Here's how the part is built. I have some questions about the finished solid (model axes, mm). Face numbers are marked on the shaded views. A direction names the side the tool comes from. Round coordinates to 2 decimals unless told otherwise and drop trailing zeros. Loops run counter-clockwise (first coordinate to the right, second up) from the corner with the lowest first, then second, coordinate; pieces in that order, holes last. Notation, with made-up numbers: (-38.5, 28.25) -> (8.5, 28.25) arc R5 ccw to (8.5, 32.25) -> close; hole circle Ø7 at (39, 11). An arc over 180 degrees is marked (long way). One line per item, written item: value. Start each with the question number.
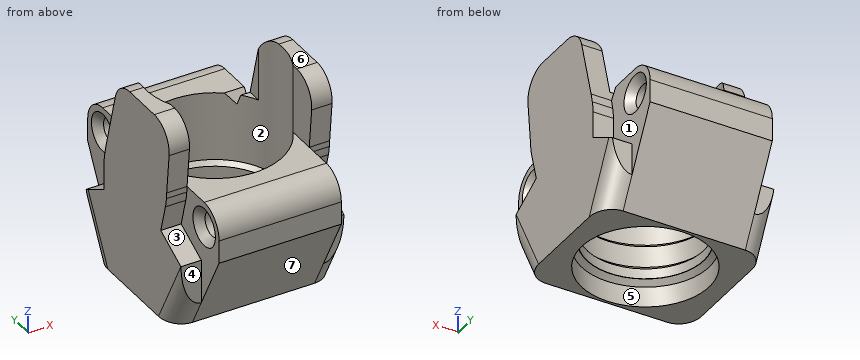
```python
from build123d import *

# Parameters (mm, degrees)
BOSS_EXTRUDE1_DEPTH           = 16
SKETCH2_W                     = 4
SKETCH2_H                     = 6.039060338
CUT_EXTRUDE1_DEPTH            = 49.391321349
FILLET1_R                     = 4
CUT_EXTRUDE2_DEPTH            = 4
SKETCH4_R                     = 12.5
CUT_EXTRUDE3_DEPTH            = 5
SKETCH5_R                     = 11.435
CUT_EXTRUDE4_DEPTH            = 45.34771704
CUT_EXTRUDE5_START            = -2
SKETCH7_R                     = 12.5
CUT_EXTRUDE5_DEPTH            = 43.347717155
CUT_EXTRUDE6_START            = 5
SKETCH8_R                     = 13.322
CUT_EXTRUDE6_DEPTH            = 38.786914196
CHAMFER5_SIZE                 = 1
SKETCH9_W                     = 24
SKETCH9_H                     = 20
CUT_EXTRUDE7_DEPTH            = 59.111966759
CSK_FOR_M4_SFHCS1_D           = 4.5
CSK_FOR_M4_SFHCS1_CSINK_D     = 7.5
CSK_FOR_M4_SFHCS1_CSINK_ANGLE = 90


with BuildPart() as part:
    # Sketch1 → Boss-Extrude1 (new, symmetric)
    with BuildSketch(Plane(origin=(0, 0, 0), x_dir=(0, 0, -1), z_dir=(1, 0, 0))):
        with BuildLine():
            Line((0, 13), (0, -13))
            Line((0, -13), (-17, -21.960950792))
            Line((-17, -21.960950792), (-21.5, -21.960950792))
            ThreePointArc((-21.5, -21.960950792), (-25.035533906, -20.496484698), (-26.5, -16.960950792))
            Line((-26.5, -16.960950792), (-26.5, -11.227190102))
            Line((-26.5, -11.227190102), (-34.5, -12.031216319))
            ThreePointArc((-34.5, -12.031216319), (-38.354100408, -10.76437729), (-39.999997516, -7.056278884))
            Line((-39.999997516, -7.056278884), (-39.999997516, 1.132402994))
            ThreePointArc((-39.999997516, 1.132402994), (-38.966764217, 4.176210139), (-36.294092741, 5.962032125))
            Line((-36.294092741, 5.962032125), (-24.512466398, 9.118909389))
            Line((-24.512466398, 9.118909389), (-26.5, 10.584515032))
            Line((-26.5, 10.584515032), (-26.5, 17.039060338))
            ThreePointArc((-26.5, 17.039060338), (-25.035533906, 20.574594244), (-21.5, 22.039060338))
            Line((-21.5, 22.039060338), (-17, 22.039060338))
            Line((-17, 22.039060338), (0, 13))
        make_face()
    extrude(amount=BOSS_EXTRUDE1_DEPTH, both=True)

    # Sketch2 → Cut-Extrude1 (cut, through all)
    with BuildSketch(Plane(origin=(0, 0, 0), x_dir=(-1, 0, 0), z_dir=(0, 0, -1))):
        with Locations((-14, 19.019530169)):
            Rectangle(SKETCH2_W, SKETCH2_H)
        with Locations((14, 19.019530169)):
            Rectangle(SKETCH2_W, SKETCH2_H)
        with Locations((14, -19.019530169)):
            Rectangle(SKETCH2_W, SKETCH2_H)
        with Locations((-14, -19.019530169)):
            Rectangle(SKETCH2_W, SKETCH2_H)
    extrude(amount=-CUT_EXTRUDE1_DEPTH, mode=Mode.SUBTRACT)

    # Fillet1
    fillet1_edges = [part.edges().sort_by_distance(p)[0] for p in [
        (16, -14.5, 2.845680173),
        (-16, -14.5, 2.845680173),
        (16, 14.5, 2.821089698),
        (-16, 14.5, 2.821089698),
    ]]
    fillet(fillet1_edges, radius=FILLET1_R)

    # Sketch3 → Cut-Extrude2 (cut)
    with BuildSketch(Plane.ZY.offset(16)):
        with BuildLine():
            Line((14.269532395, -16), (17.810147733, -9.256580566))
            Line((17.810147733, -9.256580566), (23.455857772, -10.805790893))
            ThreePointArc((23.455857772, -10.805790893), (24.367969512, -11.010765142), (25.295236814, -11.12966687))
            Line((25.295236814, -11.12966687), (26.5, -11.227190102))
            Line((26.5, -11.227190102), (26.5, -16))
            Line((26.5, -16), (14.269532395, -16))
        make_face()
        with BuildLine():
            Line((11.870259532, 16), (15.370259532, 9.753066737))
            Line((15.370259532, 9.753066737), (20.553734624, 9.753066737))
            ThreePointArc((20.553734624, 9.753066737), (21.64061559, 9.693825703), (22.714618956, 9.516804502))
            Line((22.714618956, 9.516804502), (24.512466398, 9.118909389))
            Line((24.512466398, 9.118909389), (26.5, 10.584515032))
            Line((26.5, 10.584515032), (26.5, 16))
            Line((26.5, 16), (11.870259532, 16))
        make_face()
    cut_extrude2 = extrude(amount=-CUT_EXTRUDE2_DEPTH, mode=Mode.SUBTRACT)

    # Mirror1: Cut-Extrude2 across plane
    add(cut_extrude2.mirror(Plane(origin=(0, 0, 0), x_dir=(0, 0, 1), z_dir=(1, 0, 0))), mode=Mode.SUBTRACT)

    # Sketch4 → Cut-Extrude3 (cut)
    with BuildSketch(Plane(origin=(0, 0, 0), x_dir=(-1, 0, 0), z_dir=(0, 0, -1))):
        with Locations(Location((0, 0, 0), (0, 0, 90))):
            Circle(SKETCH4_R)
    extrude(amount=-CUT_EXTRUDE3_DEPTH, mode=Mode.SUBTRACT)

    # Sketch5 → Cut-Extrude4 (cut, through all)
    with BuildSketch(Plane(origin=(0, 0, 5), x_dir=(-1, 0, 0), z_dir=(0, 0, -1))):
        with Locations(Location((0, 0, 0), (0, 0, 90))):
            Circle(SKETCH5_R)
    extrude(amount=-CUT_EXTRUDE4_DEPTH, mode=Mode.SUBTRACT)

    # Sketch7 → Cut-Extrude5 (cut, through all)
    with BuildSketch(Plane(origin=(0, 0, 5), x_dir=(-1, 0, 0), z_dir=(0, 0, -1)).offset(CUT_EXTRUDE5_START)):
        with Locations(Location((0, 0, 0), (0, 0, 90))):
            Circle(SKETCH7_R)
    extrude(amount=-CUT_EXTRUDE5_DEPTH, mode=Mode.SUBTRACT)

    # Sketch8 → Cut-Extrude6 (cut, through all)
    with BuildSketch(Plane.XY.offset(7).offset(CUT_EXTRUDE6_START)):
        with Locations(Location((0, 0, 0), (0, 0, 175.123832714))):
            Circle(SKETCH8_R)
    extrude(amount=CUT_EXTRUDE6_DEPTH, mode=Mode.SUBTRACT)

    # Chamfer5
    # the kernel refuses this chamfer: 1 mm, written as the material it adds along each edge
    with BuildSketch(Plane(origin=(0, 0, 7), x_dir=(0, 1, 0), z_dir=(-1, 0, 0))) as chamfer5_piece_1:
        Polygon((12.5 - CHAMFER5_SIZE, 0), (12.5, -CHAMFER5_SIZE), (12.5, 0), align=None)
    revolve(axis=Axis((0, 0, 7), (0, 0, -1)))
    with BuildSketch(Plane(origin=(0, 0, 5), x_dir=(0, 1, 0), z_dir=(-1, 0, 0))) as chamfer5_piece_2:
        Polygon((12.5, CHAMFER5_SIZE), (12.5 - CHAMFER5_SIZE, 0), (12.5, 0), align=None)
    revolve(axis=Axis((0, 0, 5), (0, 0, -1)))
    with BuildSketch(Plane(origin=(0, 0, 12), x_dir=(-0.9963807399610061, 0.08500247663896625, 0), z_dir=(0.08500247663896625, 0.9963807399610061, 0))) as chamfer5_piece_3_section:
        Polygon((13.322, CHAMFER5_SIZE), (13.322 - CHAMFER5_SIZE, 0), (13.322, 0), align=None)
    chamfer5_piece_3 = revolve(axis=Axis((0, 0, 12), (0, 0, 1)), mode=Mode.PRIVATE)
    chamfer5_piece_3 = chamfer5_piece_3 - Plane(origin=(0, 0, 12.578358266), x_dir=(0, 1, 0), z_dir=(0, 0, -1)) * Cylinder(12.5, 54, mode=Mode.PRIVATE)
    add(chamfer5_piece_3)

    # Sketch9 → Cut-Extrude7 (cut, through all)
    with BuildSketch(Plane(origin=(0, 17.039060338, 0), x_dir=(-1, 0, 0), z_dir=(0, 1, 0))):
        with Locations((0, 36.5)):
            Rectangle(SKETCH9_W, SKETCH9_H)
    extrude(amount=-CUT_EXTRUDE7_DEPTH, mode=Mode.SUBTRACT)

    # CSK for M4 SFHCS1 (through all)
    with Locations(Plane(origin=(12, 0, 0), x_dir=(0, 0, -1), z_dir=(1, 0, 0))):
        with Locations((-21.5, 17.039060338), (-21.5, -16.960950792)):
            csk_for_m4_sfhcs1 = CounterSinkHole(CSK_FOR_M4_SFHCS1_D / 2, CSK_FOR_M4_SFHCS1_CSINK_D / 2, counter_sink_angle=CSK_FOR_M4_SFHCS1_CSINK_ANGLE)

    # Mirror2: CSK for M4 SFHCS1 across plane
    add(csk_for_m4_sfhcs1.mirror(Plane(origin=(0, 0, 0), x_dir=(0, 0, 1), z_dir=(1, 0, 0))), mode=Mode.SUBTRACT)


solid = part.part
```
Q1. I want a section at A-A on x = 0. State how many separate pieces and enclosed holes the cut face has, plus the area to 3 significant figures.
Q2. I want a section at B-B on y = 0. Please give me the cut outline in (x, z) (3 decimals).
Q3. If we mould it in two halves opening along Y, with no side actions, what happens to the marked faces 5, 6 and 7? For each: released by +Y, released by -Y, zero draft, split by the parting line, or undercut.
Q4. I want a section at C-C on x = 14.5. Please give me the cut outline in (y, z), plus the area to 3 significant figures.
Q5. Will these pins go through, and if not, where does the flat tip stop? P1, Ø1, axis at x = 5.5, z = 16, coming from the -Y side; P2, Ø7, axis at y = -16.96, z = 21.5, coming from the -X side; P3, Ø1.2, axis at x = 15, z = 8.5, coming from the -Y side.
Q6. Which directions (+Z, -Z, +X, -X, +Y, -Y) give clear straight access to the entire face, cutting with the end or side of a thin tool? Please do the marked faces 1, 2, 3 and 4.
Q7. If I drill on line 1 along X through (y, z) = (0, 6) (3 decimals); line 2 along Y through (x, z) = (0, 23.25); line 3 along Y through (x, z) = (8, 22), over which ranges is the centre line in solid material (lowest first)?
Answers below:
1. separate pieces: 2
1. enclosed holes: 2
1. area: 291 mm^2
2. outline: (-16, 0) -> (-12.5, 0) -> (-12.5, 4) -> (-11.5, 5) -> (-11.435, 5) -> (-11.435, 7) -> (-11.5, 7) -> (-12.5, 8) -> (-12.5, 12.178) -> (-13.322, 13) -> (-13.322, 40) -> (-16, 40) -> close; (11.435, 5) -> (11.5, 5) -> (12.5, 4) -> (12.5, 0) -> (16, 0) -> (16, 40) -> (13.322, 40) -> (13.322, 13) -> (12.5, 12.178) -> (12.5, 8) -> (11.5, 7) -> (11.435, 7) -> close
3. face 5: undercut
3. face 6: zero draft
3. face 7: released by -Y
4. outline: (-16, 7.57) -> (-12.01, 0) -> (12.01, 0) -> (16, 7.51) -> (16, 11.87) -> (9.75, 15.37) -> (9.75, 20.55) arc R10 ccw to (9.52, 22.71) -> (9.12, 24.51) -> (5.96, 36.29) arc R5 ccw to (1.13, 40) -> (-7.06, 40) arc R5 ccw to (-12.03, 34.5) -> (-11.23, 26.5) -> (-11.13, 25.3) arc R10 ccw to (-10.81, 23.46) -> (-9.26, 17.81) -> (-16, 14.27) -> close
4. area: 917 mm^2
5. P1: stops at y = -21.7
5. P2: stops at x = -11.75
5. P3: stops at y = -16
6. face 1: +Z, +X, +Y
6. face 2: +Z
6. face 3: -X, -Y
6. face 4: +Z, -Z, -X, -Y
7. line 1: x = -16 to -11.435, 11.435 to 16
7. line 2: y = -21.64 to -18.38, -15.55 to -13.32, 13.32 to 15.62, 18.45 to 21.72
7. line 3: y = -21.94 to -19.15, -14.77 to -10.65, 10.65 to 14.85, 19.23 to 22.01
